```python
from build123d import *

# Parameters (mm, degrees)
SKETCH1_R               = 15
GEAR_BLANK_DEPTH        = 4
FRONT_GEAR_CHAMFER_SIZE = 2
REAR_GEAR_CHAMFER_SIZE  = 0.75
TOOTH_CUT_DEPTH         = 4
TOOTH_COPIES_COUNT      = 9
SKETCH3_R               = 4.7
BOSS_EXTRUDE1_DEPTH     = 1.54
SKETCH4_R               = 2.625
CUT_EXTRUDE1_DEPTH      = 10


with BuildPart() as part:
    # Sketch1 → Gear Blank (new body, symmetric)
    with BuildSketch(Plane.XY):
        Circle(SKETCH1_R)
    extrude(amount=GEAR_BLANK_DEPTH, both=True)

    # Front Gear Chamfer
    front_gear_chamfer_edges = [part.edges().sort_by_distance(p)[0] for p in [
        (-15, 0, 4),
    ]]
    chamfer(front_gear_chamfer_edges, length=FRONT_GEAR_CHAMFER_SIZE)

    # Rear Gear Chamfer
    rear_gear_chamfer_edges = [part.edges().sort_by_distance(p)[0] for p in [
        (-15, 0, -4),
    ]]
    chamfer(rear_gear_chamfer_edges, length=REAR_GEAR_CHAMFER_SIZE)

    # Sketch2 → Tooth Cut (cut, symmetric)
    with BuildSketch(Plane.XY):
        with BuildLine():
            ThreePointArc((3.882278974, 14.48888919), (-6.939e-06, 15), (-3.882292379, 14.488885598))
            ThreePointArc((-3.882292379, 14.488885598), (-2.012616773, 12.297020546), (-0.845415175, 9.66308818))
            ThreePointArc((-0.845415175, 9.66308818), (-4.487e-06, 9.7), (0.845406235, 9.663088963))
            ThreePointArc((0.845406235, 9.663088963), (2.012605396, 12.297022408), (3.882278974, 14.48888919))
        make_face()
    tooth_cut = extrude(amount=TOOTH_CUT_DEPTH, both=True, mode=Mode.SUBTRACT)

    # Tooth Copies: Tooth Cut ×9 about axis
    tooth_copies_axis = Axis((0, 0, 0), (0, 0, 1))
    for i in range(1, TOOTH_COPIES_COUNT):
        add(tooth_cut.rotate(tooth_copies_axis, i * 360 / TOOTH_COPIES_COUNT), mode=Mode.SUBTRACT)

    # Sketch3 → Boss-Extrude1 (add)
    with BuildSketch(Plane.XY.offset(4)):
        Circle(SKETCH3_R)
    extrude(amount=BOSS_EXTRUDE1_DEPTH)

    # Sketch4 → Cut-Extrude1 (cut)
    with BuildSketch(Plane(origin=(0, 0, -4), x_dir=(-1, 0, 0), z_dir=(0, 0, -1))):
        Circle(SKETCH4_R)
    extrude(amount=-CUT_EXTRUDE1_DEPTH, mode=Mode.SUBTRACT)


solid = part.part
```
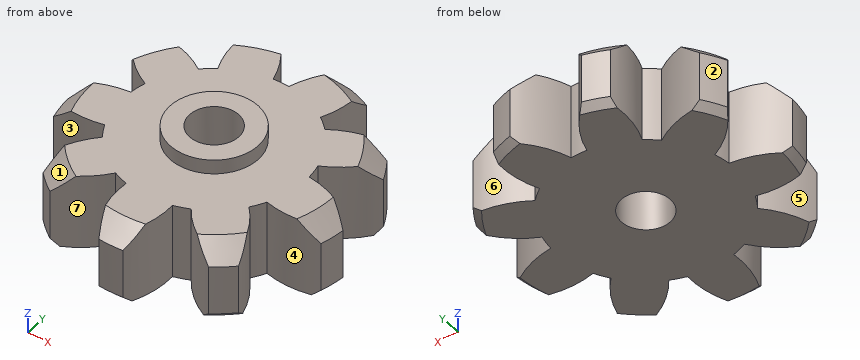
Geometry check sheet. Reference: the model listing, model coordinates, mm. Face numbers are marked on the shaded views. A direction names the side the tool comes from. Coordinates: 2 decimals unless noted, no trailing zeros. Order: outer loops, then holes, each group sorted by start corner. A loop starts at its lowest first (then second) coordinate and runs counter-clockwise, first axis right, second up. Notation, with made-up numbers: (15.5, 46) - (21.5, 46) arc R24 ccw to (21.5, 84) - close; hole circle Ø6 at (1.25, 57.5). An arc over 180 degrees is marked (long way). Answer as a JSON object with one key per item and string values. Group by question number.
Item 1: Scan lines: probe 1 along Y at (x, z) = (0, 1) (3 decimals); probe 2 along X at (y, z) = (-12, -0.75); probe 3 along X at (y, z) = (11.75, -2.5). Record each from-to range of solid material in increasing order.
Item 2: Tool access check on the marked faces 4, 5, 6 and 7. Record the directions out of +Z, -Z, +X, -X, +Y, -Y that give a thin tool (end or side, any length) a straight path to the whole face; none if there is none.
Item 3: Draft check along Y on the marked faces 1, 2 and 3. Enter one of: +Y half, -Y half, draft (parallel to the pull), parting line (faces both ways), or undercut.
Item 4: Sectioned sample at A-A, the plane x = 0. Record the cut outline in (y, z) (3 decimals), and give its area (3 significant figures).
Item 5: Depth check by flat-ended pin: pin 1 Ø2 at (x, y) = (1, 10.5) entering from +Z. Enter the tip coordinate at first touch or a pass-through.
Item 6: Sectioned sample at B-B, the plane z = 5. Record the cut outline in (x, y) (3 decimals).
Resolved:
{
 "1": {"probe 1": "-15 to -2.625, 2.625 to 9.7", "probe 2": "-9 to -7.94, -2.36 to 2.36, 7.94 to 9", "probe 3": "-6.45 to -1.69, 1.69 to 6.45"},
 "2": {"face 4": "+Z, -Z", "face 5": "+Z, -Z, -X", "face 6": "+Z, -Z, +Y", "face 7": "+Z, -Z, -Y"},
 "3": {"face 1": "-Y half", "face 2": "+Y half", "face 3": "undercut"},
 "4": {"outline": "(-15, -3.25) - (-14.25, -4) - (-2.625, -4) - (-2.625, 5.54) - (-4.7, 5.54) - (-4.7, 4) - (-13, 4) - (-15, 2) - close; (2.625, -4) - (9.7, -4) - (9.7, 4) - (4.7, 4) - (4.7, 5.54) - (2.625, 5.54) - close", "area": "160 mm^2"},
 "5": {"pin 1": "z = 4"},
 "6": {"outline": "circle Ø9.4 at (0, 0); hole circle Ø5.25 at (0, 0)"}
}
